The listing builds one solid part. Answer for the finished solid, in the listing's coordinates (mm). Round coordinates to 2 decimals unless told otherwise and drop trailing zeros. Write each loop counter-clockwise with the first axis right and the second up, starting at its lowest first coordinate (ties: lowest second). Pieces come first, ordered by that corner, then holes. Notation, with made-up numbers: M 39,19 L 82,19 A30 cw 82,41 Z; hole C 28.5,4.5 d2. An arc over 180 degrees is marked long. Put each result on its own line as item: value. Start each with the question number.
Autodesk Inventor part; units mm, degrees
ref_plane "РабПлоскость1" through (-327.803629, 8.784154, 215.836479) normal (0, 0, 1) x (1, 0, 0)
ref_plane "РабПлоскость2" through (-327.498735, 8.403036, 292.836479) normal (0, 0, -1) x (-0.999864, -0.0164918, 0)
ref_plane "РабПлоскость3" through (-672.954973, 50.067364, -86.377936) normal (-0.0164918, 0.999864, 0) x (0, 0, 1)
ref_plane "РабПлоскость1" through (-327.803629, 8.784154, 215.836479) normal (0, 0, 1) x (1, 0, 0)
sketch "Эскиз1" plane through (-327.803629, 8.784154, 215.836479) normal (0, 0, 1) x (1, 0, 0)
  line L0 (3.114831, 11.166777) -> (2.944416, 21.498705)
  line L1 (2.944416, 21.498705) -> (-3.054768, 21.399754)
  line L2 (-3.054768, 21.399754) -> (-2.884353, 11.067826)
  line L3 (-2.884353, 11.067826) -> (3.114831, 11.166777)
  line L4 (-3.393221, 41.919489) -> (-3.225183, 31.731682)
  line L5 (2.774001, 31.830633) -> (2.605963, 42.01844)
  line L6 (-3.225183, 31.731682) -> (2.774001, 31.830633)
  line L7 (2.605963, 42.01844) -> (-3.393221, 41.919489)
  line L8 (2.774001, 31.830633) -> (2.605963, 42.01844) construction
  line L9 (-3.393221, 41.919489) -> (-3.225183, 31.731682) construction
  line L10 (3.114831, 11.166777) -> (2.944416, 21.498705) construction
  line L11 (-3.054768, 21.399754) -> (-2.884353, 11.067826) construction
  line L12 (6.149374, 48.077701) -> (19.433282, 48.296806) construction
  line L13 (2.605963, 42.01844) -> (6.248325, 42.078517) construction
  point P0 (327.803629, -8.784154)
  dimension "d16" = 6
extrude "Выдавливание1" add sketch "Эскиз1" against normal blind 6
ref_plane "РабПлоскость2" through (-327.498735, 8.403036, 292.836479) normal (0, 0, -1) x (-0.999864, -0.0164918, 0)
sketch "Эскиз2" plane through (-327.498735, 8.403036, 292.836479) normal (0, 0, -1) x (-0.999864, -0.0164918, 0)
  line L0 (-3, 21.833317) -> (3, 21.833317)
  line L1 (3, 21.833317) -> (3, 11.499984)
  line L2 (3, 11.5) -> (-3, 11.5)
  line L3 (-3, 11.499984) -> (-3, 21.833317)
  line L4 (3, 32.16665) -> (-3, 32.16665)
  line L5 (-3, 32.16665) -> (-3, 42.355843)
  line L6 (-3, 42.5) -> (3, 42.5)
  line L7 (3, 42.355843) -> (3, 32.16665)
  line L8 (-3, 11.499984) -> (-3, 21.833317) construction
  line L9 (3, 21.833317) -> (3, 11.499984) construction
  line L10 (-3, 32.16665) -> (-3, 42.355843) construction
  line L11 (3, 42.355843) -> (3, 32.16665) construction
  point P0 (-327.315615, -13.802923)
sketch "Эскиз2 outline for Выдавливание2" plane through (-327.498735, 8.403036, 292.836479) normal (0, 0, -1) x (-0.999864, -0.0164918, 0)
  line L0 (3, 32.16665) -> (3, 42.355843)
  line L1 (-3, 32.16665) -> (3, 32.16665)
  line L2 (-3, 42.355843) -> (-3, 32.16665)
  line L3 (3, 42.355843) -> (-3, 42.355843)
  line L4 (-3, 21.833317) -> (-3, 11.499984)
  line L5 (3, 21.833317) -> (-3, 21.833317)
  line L6 (3, 11.499984) -> (3, 21.833317)
  line L7 (-3, 11.499984) -> (3, 11.499984)
extrude "Выдавливание2" add sketch "Эскиз2 outline for Выдавливание2" against normal blind 6
sketch "Эскиз3" plane through (-327.498735, 8.403036, 292.836479) normal (0, 0, -1) x (-0.999864, -0.0164918, 0)
  line L0 (6.642857, 42.355843) -> (3, 42.355843)
  line L1 (-3, 32.166667) -> (-3, 21.833333)
  line L2 (-3, 21.833333) -> (3, 21.833333)
  line L3 (3, 21.833333) -> (3, 32.166667)
  line L4 (3, 32.166667) -> (-3, 32.166667)
  line L5 (-3, 42.355843) -> (3, 42.355843)
  line L6 (3, 42.355843) -> (3, 11.495073)
  line L7 (3, 11.495073) -> (-3, 11.495073)
  line L8 (-3, 11.495073) -> (-3, 42.355843)
  point P0 (-327.315615, -13.802923)
  point P1 (-3, 21.833333)
  point P2 (3, 21.833333)
  point P3 (3, 42.355843)
extrude "Выдавливание3" add sketch "Эскиз3" along normal up to surface (77 mm away)
sketch "Эскиз4" plane through (-331.19685, 50.703643, 209.836479) normal (-0.999864, -0.0164918, 0) x (0, 0, 1)
  line L0 (0, -14) -> (6, -14) construction
  line L1 (0, -17) -> (6, -17) construction
  line L2 (6, -17) -> (6, -14)
  line L3 (6, -14) -> (12.35, -14)
  line L4 (12.35, -14) -> (12.35, -12.75)
  line L5 (12.35, -12.75) -> (14.65, -12.75)
  line L6 (14.65, -12.75) -> (14.65, -14)
  line L7 (14.65, -14) -> (21, -14)
  line L8 (21, -14) -> (21, -17)
  line L9 (21, -17) -> (14.65, -17)
  line L10 (14.65, -17) -> (14.65, -18.25)
  line L11 (14.65, -18.25) -> (12.35, -18.25)
  line L12 (12.35, -18.25) -> (12.35, -17)
  line L13 (12.35, -17) -> (6, -17)
  line L14 (0, -20.522506) -> (0, -30.855843) construction
  line L15 (89, -10.189193) -> (89, 0) construction
  line L16 (0, -30.855843) -> (89, 0) construction
  line L17 (44.5, 0) -> (44.5, -30.855843) construction
  line L18 (89, -14) -> (83, -14) construction
  line L19 (89, -17) -> (83, -17) construction
  line L20 (83, -17) -> (83, -14)
  line L21 (83, -14) -> (76.65, -14)
  line L22 (76.65, -14) -> (76.65, -12.75)
  line L23 (76.65, -12.75) -> (74.35, -12.75)
  line L24 (74.35, -12.75) -> (74.35, -14)
  line L25 (74.35, -14) -> (68, -14)
  line L26 (68, -14) -> (68, -17)
  line L27 (68, -17) -> (74.35, -17)
  line L28 (74.35, -17) -> (74.35, -18.25)
  line L29 (74.35, -18.25) -> (76.65, -18.25)
  line L30 (76.65, -18.25) -> (76.65, -17)
  line L31 (76.65, -17) -> (83, -17)
  point P0 (-209.836479, -56.158766)
  point P1 (44.5, -15.427922)
  dimension "d9" = 2.3
  dimension "d10" = 5.5
  dimension "d11" = 15
extrude "Выдавливание4" cut sketch "Эскиз4" against normal blind 6
ref_plane "РабПлоскость3" through (-672.954973, 50.067364, -86.377936) normal (-0.0164918, 0.999864, 0) x (0, 0, 1)
sketch "Эскиз6" plane through (-325.197666, 50.802594, 298.836479) normal (-0.0164918, 0.999864, 0) x (0.999864, 0.0164918, 0)
  line L0 (-6, 89) -> (-6, 0) construction
  line L1 (0, 0) -> (0, 89) construction
  line L2 (-6, 32) -> (0, 32)
  line L3 (0, 32) -> (0, 57)
  line L4 (0, 57) -> (-6, 57)
  line L5 (-6, 57) -> (-6, 32)
  line L6 (0, 89) -> (-6, 89)
  line L7 (-3, 89) -> (-3, 57) construction
  line L8 (-3, 32) -> (-3, 0) construction
  line L9 (0, 0) -> (-6, 0)
  point P0 (324.315615, 298.836479)
  dimension "d17" = 25
extrude "Выдавливание6" add sketch "Эскиз6" along normal blind 6
equation "\"d1\" = d0"
equation "\"d3\" = d0"
equation "\"d7\" = d0"
equation "\"d12\" = d3"
equation "\"d0\" = d16"
properties part number "motor1"
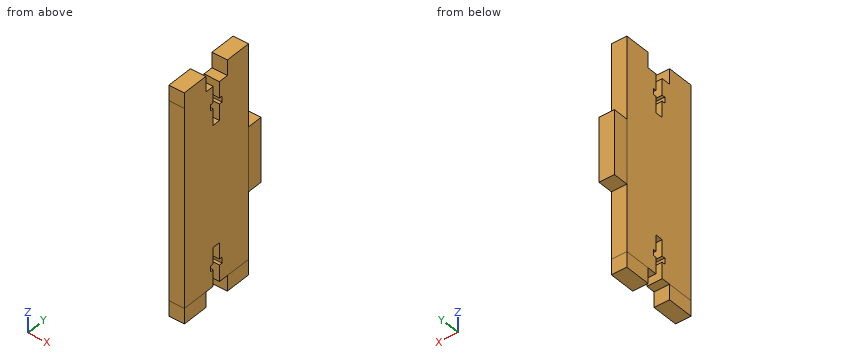
Item 1: Consider line 1 along Y through (x, z) = (-325.25, 214.5); line 2 along X through (y, z) = (30.5, 269); line 3 along Y through (x, z) = (-325.75, 235). Determine where each line is inside the solid, lowest interval first. Write a range as [from, to].
Item 2: Section C-C (z = 252.5) is taken. Give the vertices of the cut face in (x, y).
Item 3: Section B-B (y = 44.5) is taken. Give the vertices of the cut face in (x, z).
Item 4: Section D-D (z = 240) is taken. Give the vertices of the cut face in (x, y), and give its area (3 significant figures).
Item 5: Section A-A (z = 282) is taken. Give the vertices of the cut face in (x, y).
Item 6: Flat-ended cylindrical pins translate along their axes: pin 1 (1.1 mm diameter, centred on x = -328.5, y = 31.5, fed in from +Z); pin 2 (6 mm diameter, centred on y = 26.5, z = 260.5, fed in from +X); pin 3 (4 mm diameter, centred on y = 26.5, z = 270, fed in from -X). Find the tip coordinate at first contact, or state that the pin passes through.
Output values:
1. line 1: y = [19.94, 30.28], [40.61, 50.8]
1. line 2: x = [-330.86, -324.86]
1. line 3: y = [19.93, 50.79]
2. outline: M -331.3,56.7 L -330.69,19.85 L -324.69,19.95 L -325.3,56.8 Z
3. outline: M -331.09,209.84 L -325.09,209.84 L -325.09,298.84 L -331.09,298.84 Z
4. outline: M -331.2,50.7 L -330.69,19.85 L -324.69,19.95 L -325.2,50.8 Z
4. area: 185 mm^2
5. outline: M -331.2,50.7 L -330.97,36.71 L -324.97,36.8 L -325.2,50.8 Z; M -330.92,33.71 L -330.69,19.85 L -324.69,19.95 L -324.92,33.8 Z
6. pin 1: stops at z = 292.84
6. pin 2: stops at x = -324.75
6. pin 3: stops at x = -330.83
